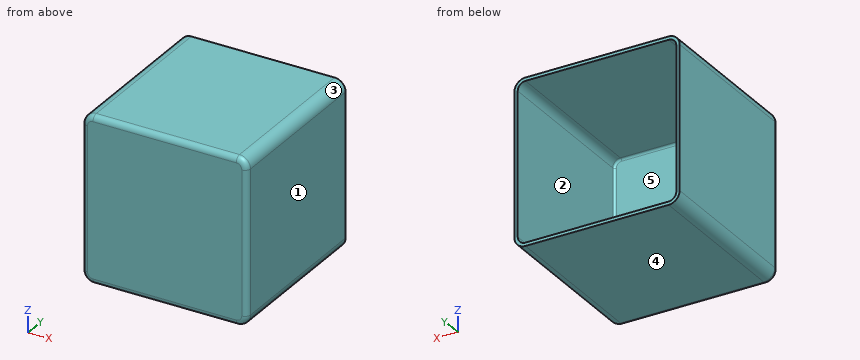
```python
from build123d import *

# Parameters (mm, degrees)
CROQUIS1_W     = 150
CROQUIS1_H     = 150
EXTRUIR1_DEPTH = 150
REDONDEO1_R    = 10
REDONDEO2_R    = 5
VACIADO1_T     = -3


with BuildPart() as part:
    # Croquis1 → Extruir1 (new body)
    with BuildSketch(Plane(origin=(0, 0, 0), x_dir=(1, 0, 0), z_dir=(0, 1, 0))):
        Rectangle(CROQUIS1_W, CROQUIS1_H)
    extrude(amount=-EXTRUIR1_DEPTH)

    # Redondeo1
    redondeo1_edges = [part.edges().sort_by_distance(p)[0] for p in [
        (-75, -75, -75),
        (75, -75, -75),
        (75, -75, 75),
        (-75, -75, 75),
    ]]
    fillet(redondeo1_edges, radius=REDONDEO1_R)

    # Redondeo2
    redondeo2_edges = [part.edges().sort_by_distance(p)[0] for p in [
        (-75, -150, 0),
        (0, -150, 75),
        (0, -150, -75),
        (75, -150, 0),
        (72.071067812, -150, -72.071067812),
        (72.071067812, -150, 72.071067812),
        (-72.071067812, -150, -72.071067812),
        (-72.071067812, -150, 72.071067812),
    ]]
    fillet(redondeo2_edges, radius=REDONDEO2_R)

    # Vaciado1
    vaciado1_openings = [part.faces().sort_by_distance(p)[0] for p in [
        (0, 0, 0),
    ]]
    offset(amount=VACIADO1_T, openings=vaciado1_openings, kind=Kind.INTERSECTION)


solid = part.part
```
Check sheet for the modelled part. Datum: model origin and axes. Units: mm. Face numbers are marked on the shaded views. A direction names the side the tool comes from. Round coordinates to 2 decimals unless told otherwise and drop trailing zeros. Order: outer loops, then holes, each group sorted by start corner. A loop starts at its lowest first (then second) coordinate and runs counter-clockwise, first axis right, second up.
1) Section check A-A (x = -61). Record the boundary of the cut face in (y, z).
2) Section check B-B (z = 51.5). Record the boundary of the cut face in (x, y).
3) Section check C-C (y = -19.5). Record the boundary of the cut face in (x, z).
4) Tool access check on the marked faces 1 and 2. Record the directions out of +Z, -Z, +X, -X, +Y, -Y that give a thin tool (end or side, any length) a straight path to the whole face; none if there is none.
5) Go/stop test with a flat-tipped pin: pin 1 Ø8 at (x, z) = (-31, 60) entering from +Y. Record where the tip stops, or that it passes through.
6) Mould release check, pull along Z, two halves, no side actions. Record for the marked faces 3, 4 and 5: +Z half, -Z half, draft (parallel to the pull), parting line (faces both ways), or undercut.
7) Scan lines: line 1 (Z direction, x = -18.5, y = -19); line 2 (Y direction, x = -61.5, z = -22.5). Record each from-to range of solid material in increasing order.
Result:
1. outline: (-150, -70) arc R5 ccw to (-145, -75) - (0, -75) - (0, -72) - (-145, -72) arc R2 cw to (-147, -70) - (-147, 70) arc R2 cw to (-145, 72) - (0, 72) - (0, 75) - (-145, 75) arc R5 ccw to (-150, 70) - close
2. outline: (-75, -145) arc R5 ccw to (-70, -150) - (70, -150) arc R5 ccw to (75, -145) - (75, 0) - (72, 0) - (72, -145) arc R2 cw to (70, -147) - (-70, -147) arc R2 cw to (-72, -145) - (-72, 0) - (-75, 0) - close
3. outline: (-75, -65) arc R10 ccw to (-65, -75) - (65, -75) arc R10 ccw to (75, -65) - (75, 65) arc R10 ccw to (65, 75) - (-65, 75) arc R10 ccw to (-75, 65) - close; hole (-72, -65) arc R7 ccw to (-65, -72) - (65, -72) arc R7 ccw to (72, -65) - (72, 65) arc R7 ccw to (65, 72) - (-65, 72) arc R7 ccw to (-72, 65) - close
4. face 1: +Z, -Z, +X, +Y, -Y
4. face 2: +Y
5. pin 1: stops at y = -147
6. face 3: +Z half
6. face 4: -Z half
6. face 5: undercut
7. line 1: z = -75 to -72, 72 to 75
7. line 2: y = -150 to -147
